Part print with two shaded views. Sizes in mm from the minimum x, y, z corner. A direction names the side the tool comes from. Coordinates: 2 decimals unless noted, no trailing zeros. Loops run counter-clockwise (first coordinate to the right, second up) from the corner with the lowest first, then second, coordinate; pieces in that order, holes last. Notation, with made-up numbers: M -30.5,-30 L 8.5,-30 A17 cw 8.5,-1 Z; hole C 15,50.5 d8. An arc over 180 degrees is marked long. Write item = value, one per line. Start each with the question number.
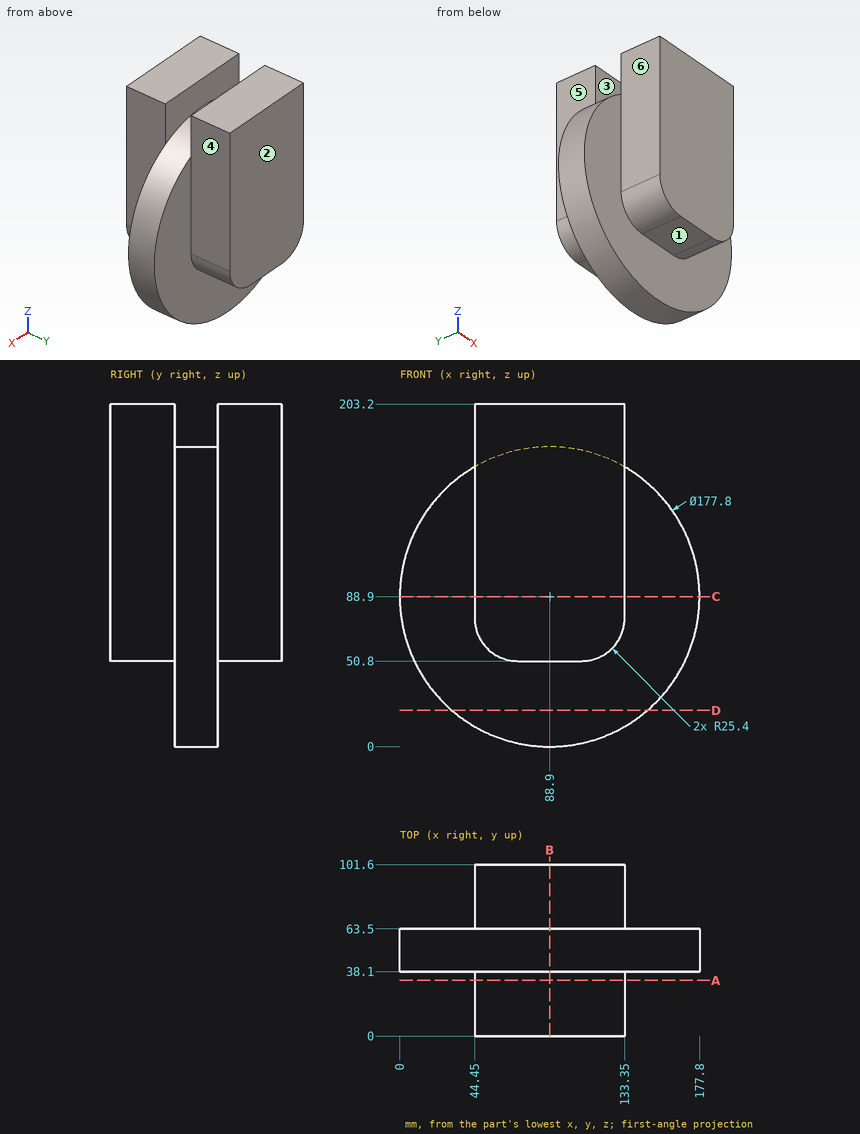
Item 1: Pin check, flat tips, straight feed: pin 1 Ø12 at (y, z) = (17.5, 122.5) entering from +X; pin 2 Ø1.5 at (y, z) = (29, 65) entering from -X; pin 3 Ø1 at (x, y) = (121.5, 52.5) entering from +Z. Stop position of each tip, or through.
Item 2: Cut at B-B (x = 88.9). Give the cut face in (y, z), plus the area to 3 significant figures.
Item 3: Probe L1, parallel to Y at x = 152, z = 49; L2, parallel to Y at x = 131, z = 168.5; L3, parallel to X at y = 78, z = 78.5. List the from-to ranges inside material, lowest first.
Item 4: Pull direction Y, two halves, no side cores. Call the marked faces 1, 2 and 3: +Y half, -Y half, draft (parallel to the pull), parting line (faces both ways), or undercut.
Item 5: 3-axis set-ups, long thin cutter, end or side, ignore diameter. For the marked faces 4, 5 and 6: which of +Z, -Z, +X, -X, +Y, -Y reach the whole face in a straight line?
Item 6: Cut at C-C (z = 88.9). Give the cut face in (x, y).
Item 7: Cut at D-D (z = 21.5). Give the cut face in (x, y), plus the area to 3 significant figures.
Item 8: Cut at A-A (y = 33). Give the cut face in (x, z), plus the area to 3 significant figures.
Reported:
q1.pin_1 = 133.35
q1.pin_2 = 46.7
q1.pin_3 = 171.8
q2.outline = M 0,50.8 L 38.1,50.8 L 38.1,0 L 63.5,0 L 63.5,50.8 L 101.6,50.8 L 101.6,203.2 L 63.5,203.2 L 63.5,177.8 L 38.1,177.8 L 38.1,203.2 L 0,203.2 Z
q2.area = 16,100 mm^2
q3.L1 = 38.1 to 63.5
q3.L2 = 0 to 38.1, 63.5 to 101.6
q3.L3 = 44.45 to 133.35
q4.face_1 = draft
q4.face_2 = +Y half
q4.face_3 = undercut
q5.face_4 = +Z, -Z, +X, +Y
q5.face_5 = +Z, -Z, -X, +Y
q5.face_6 = +Z, -Z, -X, -Y
q6.outline = M 0,38.1 L 44.45,38.1 L 44.45,0 L 133.35,0 L 133.35,38.1 L 177.8,38.1 L 177.8,63.5 L 133.35,63.5 L 133.35,101.6 L 44.45,101.6 L 44.45,63.5 L 0,63.5 Z
q7.outline = M 30.93,38.1 L 146.87,38.1 L 146.87,63.5 L 30.93,63.5 Z
q7.area = 2,940 mm^2
q8.outline = M 44.45,76.2 A25.4 ccw 69.85,50.8 L 107.95,50.8 A25.4 ccw 133.35,76.2 L 133.35,203.2 L 44.45,203.2 Z
q8.area = 13,300 mm^2
